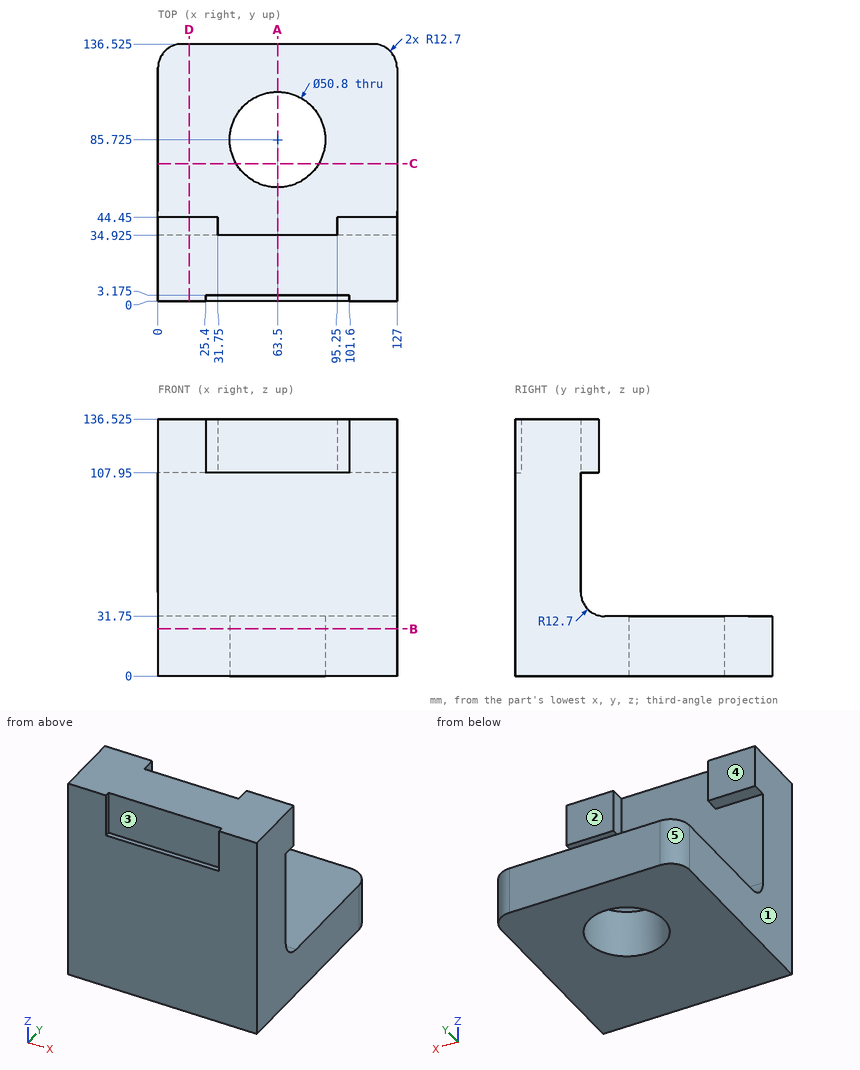
Study the drawing (mm; zero at the part's minimum x, y, z) and answer. A direction names the side the tool comes from. Coordinates: 2 decimals unless noted, no trailing zeros. Write each loop counter-clockwise with the first axis right and the second up, starting at its lowest first coordinate (ties: lowest second). Pieces come first, ordered by that corner, then holes.
Q1. A cutting plane is placed at B-B, the plane z = 25. Give the vertices of the cut face in (x, y) (3 decimals), then the cut area to 3 significant figures.
Q2. Determine the mould class of the marked faces 1, 2 and 3 for opening direction X: released by +X, released by -X, zero draft, split by the parting line, or undercut.
Q3. Find the intervals of material crossed by line 1 (X direction, y = 41, z = 130.5); line 2 (Y direction, x = 63, z = 16) (3 decimals); line 3 (Y direction, x = 114, z = 96) (3 decimals), in increasing order.
Q4. A cutting plane is placed at C-C, the plane y = 73. Give the vertices of the cut face in (x, z).
Q5. A cutting plane is placed at D-D, the plane x = 16.5. Give the vertices of the cut face in (y, z) (3 decimals), then the cut area to 3 significant figures.
Q6. A cutting plane is placed at A-A, the plane x = 63.5. Give the vertices of the cut face in (y, z) (3 decimals), then the cut area to 3 significant figures.
Q7. Which of the six approach directions +Z, -Z, +X, -X, +Y, -Y give full straight-line access (tool end or side, diameter ignored) to the marked faces 4 and 5?
Q8. Each of these flat-tipped pins is pushed along its axis until it touches: pin 1 Ø14.5 at (x, z) = (116, 123) entering from +Y; pin 2 Ø1 at (x, y) = (73, 56.5) entering from +Z; pin 3 Ø14.5 at (x, z) = (52.5, 118.5) entering from -Y (3 decimals). Where does it stop, or does it pass through?
Findings below:
1. outline: (0, 0) - (127, 0) - (127, 123.825) arc R12.7 ccw to (114.3, 136.525) - (12.7, 136.525) arc R12.7 ccw to (0, 123.825) - close; hole circle Ø50.8 at (63.5, 85.725)
1. area: 15,200 mm2
2. face 1: released by -X
2. face 2: zero draft
2. face 3: undercut
3. line 1: x = 0 to 31.75, 95.25 to 127
3. line 2: y = 0 to 60.33, 111.12 to 136.525
3. line 3: y = 0 to 34.925
4. outline: (0, 0) - (41.52, 0) - (41.52, 31.75) - (0, 31.75) - close; (85.48, 0) - (127, 0) - (127, 31.75) - (85.48, 31.75) - close
5. outline: (0, 0) - (136.525, 0) - (136.525, 31.75) - (47.625, 31.75) arc R12.7 cw to (34.925, 44.45) - (34.925, 107.95) - (44.45, 107.95) - (44.45, 136.525) - (0, 136.525) - close
5. area: 8,300 mm2
6. outline: (0, 0) - (60.325, 0) - (60.325, 31.75) - (47.625, 31.75) arc R12.7 cw to (34.925, 44.45) - (34.925, 136.525) - (3.175, 136.525) - (3.175, 107.95) - (0, 107.95) - close; (111.125, 0) - (136.525, 0) - (136.525, 31.75) - (111.125, 31.75) - close
6. area: 6,320 mm2
7. face 4: +Z, +X, -X, +Y
7. face 5: +Z, -Z, -X, +Y
8. pin 1: stops at y = 44.45
8. pin 2: stops at z = 31.75
8. pin 3: stops at y = 3.175
